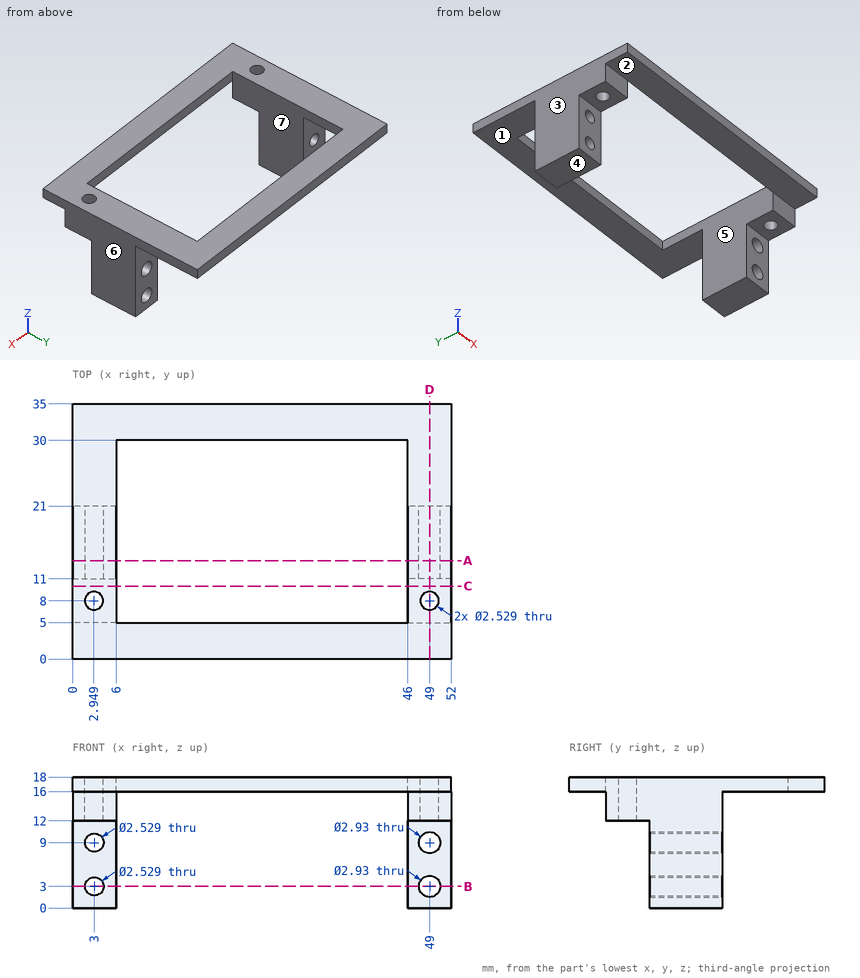
Input: dimensioned drawing with shaded views. Units: mm. Origin: part minimum x, y, z. A direction names the side the tool comes from. Round coordinates to 2 decimals unless told otherwise and drop trailing zeros. Loops run counter-clockwise (first coordinate to the right, second up) from the corner with the lowest first, then second, coordinate; pieces in that order, holes last. Notation, with made-up numbers: (4.5, 70.5) -> (35.5, 70.5) arc R29 cw to (35.5, 91.5) -> close; hole circle Ø11 at (3, 85.25). An arc over 180 degrees is marked (long way). Use one line per item in the form item = value. Start each with the question number.
1) Line query: L1, parallel to X at y = 16.75, z = 3 (1 decimal); L2, parallel to Z at x = 49, y = 13 (3 decimals); L3, parallel to Z at x = 3, y = 19. Output: solid intervals per line, ascending.
2) Access query for the marked faces 1, 2 and 3. Directions: +Z, -Z, +X, -X, +Y, -Y. A direction counts if a zero-diameter tool reaches every point of the face in a straight line with its end or side. Return the directions, or none.
3) First-contact query: P1, Ø1.2, axis at x = 1.5, z = 13.5, coming from the -Y side; P2, Ø5.5, axis at x = 20.5, y = 3, coming from the -Z side; P3, Ø5, axis at x = 2.5, z = 8.5, coming from the +Y side. Flat tips, straight axial feed; report the tip coordinate or a pass-through.
4) Section C-C on y = 10. Output: boundary loops of the cut face in (x, z).
5) Draft query along X for the marked faces 4, 5, 6 and 7. Return one class per face: released by +X, released by -X, zero draft, split by the parting line, or undercut.
6) Section B-B on z = 3. Output: boundary loops of the cut face in (x, y) (1 decimal).
7) Section D-D on x = 49. Output: boundary loops of the cut face in (y, z) (1 decimal).
8) Section A-A on y = 13.5. Output: boundary loops of the cut face in (x, z) (1 decimal), then the cut area to 3 significant figures.
Response:
q1.L1 = 0 to 1.7, 4.3 to 6, 46 to 47.5, 50.5 to 52
q1.L2 = 0 to 1.535, 4.465 to 7.535, 10.465 to 18
q1.L3 = 0 to 1.74, 4.26 to 7.74, 10.26 to 18
q2.face_1 = -Z, +X, -X, +Y
q2.face_2 = -Z, +X, -X, -Y
q2.face_3 = +Z, -Z, -X, +Y, -Y
q3.P1 = 5
q3.P2 = 16
q3.P3 = 21
q4.outline = (0, 12) -> (6, 12) -> (6, 18) -> (0, 18) -> close; (46, 12) -> (52, 12) -> (52, 18) -> (46, 18) -> close
q5.face_4 = zero draft
q5.face_5 = undercut
q5.face_6 = released by +X
q5.face_7 = undercut
q6.outline = (0, 11) -> (1.7, 11) -> (1.7, 21) -> (0, 21) -> close; (4.3, 11) -> (6, 11) -> (6, 21) -> (4.3, 21) -> close; (46, 11) -> (47.5, 11) -> (47.5, 21) -> (46, 21) -> close; (50.5, 11) -> (52, 11) -> (52, 21) -> (50.5, 21) -> close
q7.outline = (0, 16) -> (5, 16) -> (5, 12) -> (6.7, 12) -> (6.7, 18) -> (0, 18) -> close; (9.3, 12) -> (11, 12) -> (11, 10.5) -> (21, 10.5) -> (21, 16) -> (35, 16) -> (35, 18) -> (9.3, 18) -> close; (11, 0) -> (21, 0) -> (21, 1.5) -> (11, 1.5) -> close; (11, 4.5) -> (21, 4.5) -> (21, 7.5) -> (11, 7.5) -> close
q8.outline = (0, 0) -> (6, 0) -> (6, 18) -> (0, 18) -> close; (46, 0) -> (52, 0) -> (52, 18) -> (46, 18) -> close; hole circle Ø2.5 at (3, 3); hole circle Ø2.5 at (3, 9); hole circle Ø2.9 at (49, 3); hole circle Ø2.9 at (49, 9)
q8.area = 192 mm^2
